Read the model definition and answer for the solid it produces. Units are mm, in the model's axes. Face numbers are marked on the shaded views. A direction names the side the tool comes from. Coordinates: 2 decimals unless noted, no trailing zeros. Write each loop counter-clockwise with the first axis right and the second up, starting at its lowest first coordinate (ties: lowest second). Pieces come first, ordered by that corner, then holes. Notation, with made-up numbers: (56, 49.5) -> (104, 49.5) arc R22 ccw to (104, 69.5) -> close; hole circle Ø4 at (20, 85). An arc over 180 degrees is marked (long way). One line per item, written item: value. Start each with the question number.
1. For a pull along X with two mould halves and no side action, classify the marked faces 4, 5 and 6 as pulls with the +X half, pulls with the -X half, needs draft (parallel to the pull), parting line crosses it, or undercut.
2. Given P1, Ø3, axis at y = 3, z = 0.5, coming from the +X side; P2, Ø1.9, axis at x = 0.5, y = -2, coming from the +Z side; P3, Ø2, axis at y = 6.5, z = -1.5, coming from the -X side, each flat-ended and moving along its own axis, determine where each tip first touches the part or whether it passes through.
3. Find section D-D, the plane y = 2.5. Write down the section's boundary in (x, z), and give its area (3 significant figures).
4. Find section B-B, the plane x = 0. Write down the section's boundary in (y, z), and give its area (3 significant figures).
5. Find section A-A, the plane y = -2.25. Write down the section's boundary in (x, z), and give its area (3 significant figures).
6. For the marked faces 1, 2 and 3, determine the directions among +Z, -Z, +X, -X, +Y, -Y from which every point of the face is accessible in a straight line to the end or side of a thin tool.
7. Find section C-C, the plane z = -1.25. Write down the section's boundary in (x, y), and give its area (3 significant figures).
8. Consider line 1 along Y through (x, z) = (3.75, 2.25); line 2 along Y through (x, z) = (-0.5, 0); line 3 along X through (y, z) = (3.5, 2). Determine where each line is inside the solid, lowest interval first.
```python
from build123d import *

# Parameters (mm, degrees)
SKETCH1_R           = 4.7
BOSS_EXTRUDE1_DEPTH = 2
SKETCH2_R           = 2.5
BOSS_EXTRUDE2_DEPTH = 5.6
SKETCH3_R           = 1.9
BOSS_EXTRUDE3_DEPTH = 0.4
CUT_EXTRUDE1_DEPTH  = 1.25


with BuildPart() as part:
    # Sketch1 → Boss-Extrude1 (new, symmetric)
    with BuildSketch(Plane(origin=(0, -2, 0), x_dir=(1, 0, 0), z_dir=(0, 1, 0))):
        with Locations(Location((0, 0, 0), (0, 0, 270))):
            Circle(SKETCH1_R)
    extrude(amount=BOSS_EXTRUDE1_DEPTH, both=True)

    # Sketch2 → Boss-Extrude2 (add, symmetric)
    with BuildSketch(Plane(origin=(0, 5.6, 0), x_dir=(1, 0, 0), z_dir=(0, 1, 0))):
        with Locations(Location((0, 0, 0), (0, 0, 270))):
            Circle(SKETCH2_R)
    extrude(amount=BOSS_EXTRUDE2_DEPTH, both=True)

    # Sketch3 → Boss-Extrude3 (add, symmetric)
    with BuildSketch(Plane(origin=(0, 11.6, 0), x_dir=(1, 0, 0), z_dir=(0, 1, 0))):
        with Locations(Location((0, 0, 0), (0, 0, 270))):
            Circle(SKETCH3_R)
    extrude(amount=BOSS_EXTRUDE3_DEPTH, both=True)

    # Sketch4 → Cut-Extrude1 (cut, symmetric)
    with BuildSketch(Plane(origin=(0, -2.75, 0), x_dir=(1, 0, 0), z_dir=(0, 1, 0))):
        Polygon((1.732050808, 0), (0.866025404, -1.5), (-0.866025404, -1.5), (-1.732050808, 0), (-0.866025404, 1.5), (0.866025404, 1.5), align=None)
    extrude(amount=CUT_EXTRUDE1_DEPTH, both=True, mode=Mode.SUBTRACT)


solid = part.part
```
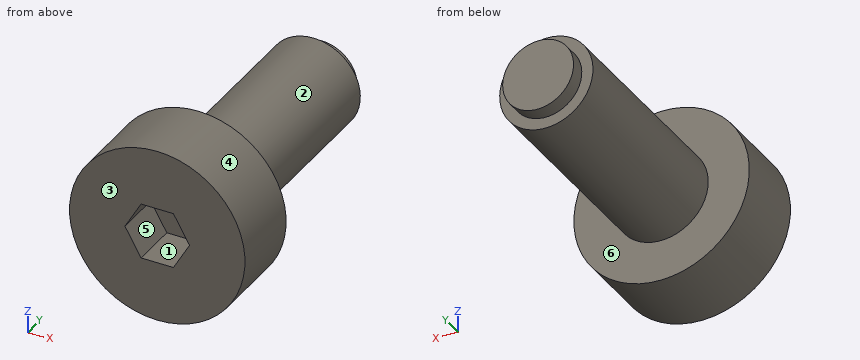
Answer block:
1. face 4: parting line crosses it
1. face 5: undercut
1. face 6: needs draft
2. P1: stops at x = 2.5
2. P2: stops at z = 4.7
2. P3: stops at x = -2.45
3. outline: circle Ø5 at (0, 0)
3. area: 19.6 mm2
4. outline: (-4, -4.7) -> (0, -4.7) -> (0, -2.5) -> (11.2, -2.5) -> (11.2, -1.9) -> (12, -1.9) -> (12, 1.9) -> (11.2, 1.9) -> (11.2, 2.5) -> (0, 2.5) -> (0, 4.7) -> (-4, 4.7) -> (-4, 1.5) -> (-1.5, 1.5) -> (-1.5, -1.5) -> (-4, -1.5) -> close
4. area: 89.1 mm2
5. outline: circle Ø9.4 at (0, 0); hole (-1.73, 0) -> (-0.87, -1.5) -> (0.87, -1.5) -> (1.73, 0) -> (0.87, 1.5) -> (-0.87, 1.5) -> close
5. area: 61.6 mm2
6. face 1: -Y
6. face 2: +Y
6. face 3: +Z, -Z, +X, -X, -Y
7. outline: (-4.53, -4) -> (-1.01, -4) -> (-1.01, -1.5) -> (1.01, -1.5) -> (1.01, -4) -> (4.53, -4) -> (4.53, 0) -> (2.17, 0) -> (2.17, 11.2) -> (1.43, 11.2) -> (1.43, 12) -> (-1.43, 12) -> (-1.43, 11.2) -> (-2.17, 11.2) -> (-2.17, 0) -> (-4.53, 0) -> close
7. area: 82.0 mm2
8. line 1: y = -4 to 0
8. line 2: y = -1.5 to 12
8. line 3: x = -1.5 to 1.5
